Autodesk Inventor part; units mm, degrees
ref_plane "YZ Plane" through (0, 0, 0) normal (1, 0, 0) x (0, 1, 0)
ref_plane "XZ Plane" through (0, 0, 0) normal (0, 1, 0) x (-1, 0, 0)
ref_plane "XY Plane" through (0, 0, 0) normal (0, 0, 1) x (1, 0, 0)
sketch "Boceto1" plane through (0, 0, 0) normal (1, 0, 0) x (0, 1, 0)
  line L0 (0.5, 9) -> (-0.5, 9)
  line L1 (-0.5, 9) -> (-0.5, -9)
  line L2 (-0.5, -9) -> (0.5, -9)
  line L3 (0.5, -9) -> (0.5, 9)
  point P0 (0, 0)
  dimension "d0" = 1
  dimension "d1" = 18
  dimension "d2" = 9
  dimension "d3" = 0.5
extrude "Extrusión1" add sketch "Boceto1" along normal blind 50
sketch "Boceto2" plane through (0, 0.5, 9) normal (0, 1, 0) x (1, 0, 0)
  line L0 (0, 0) -> (50, 0)
  line L1 (0, 18) -> (50, 18)
  line L2 (0, 18) -> (0, 0)
  line L3 (25, 0) -> (25, 18)
  line L4 (0, 0) -> (50, 0)
  point P0 (0, 9)
  point P1 (2.54, 5.19)
  point P2 (2.54, 7.73)
  point P3 (2.54, 10.27)
  point P4 (2.54, 12.81)
  point P5 (47.46, 5.19)
  point P6 (47.46, 7.73)
  point P7 (47.46, 10.27)
  point P8 (47.46, 12.81)
  dimension "d6" = 5.19
  dimension "d8" = 2.54
  dimension "d9" = 2.54
  dimension "d10" = 2.54
  dimension "d11" = 2.54
hole "Agujero1" at (2.54, 0.5, 3.81) at (2.54, 0.5, 1.27) at (2.54, 0.5, -1.27) at (2.54, 0.5, -3.81) at (25, 0.5, 9) at (25, 0.5, -9) at (47.46, 0.5, -3.81) at (47.46, 0.5, -1.27) at (47.46, 0.5, 1.27) at (47.46, 0.5, 3.81) direction (0, -1, 0) diameter 0.9 end through all
sketch "Boceto3" plane through (0, 0.5, 9) normal (0, 1, 0) x (1, 0, 0)
  line L0 (37.0371, 5) -> (41.9064, 5)
  line L1 (41.9064, 5) -> (41.9064, 13)
  line L2 (41.9064, 13) -> (37.0371, 13)
  line L3 (37.0371, 13) -> (37.0371, 5)
  line L4 (25.45, 0) -> (50, 0)
  line L5 (25.45, 18) -> (50, 18)
  point P0 (0, 9)
  dimension "d19" = 5
  dimension "d20" = 5
extrude "Extrusión2" add sketch "Boceto3" along normal blind 5
properties part number "MAX485"
Build history of the part. All positions in model axes, mm. A direction names the side the tool comes from. Coordinates: 2 decimals unless noted, no trailing zeros. Order: outer loops, then holes, each group sorted by start corner. A loop starts at its lowest first (then second) coordinate and runs counter-clockwise, first axis right, second up. Notation, with made-up numbers: (-32.5, 50) - (17.5, 50) arc R11 ccw to (17.5, 62) - close; hole circle Ø8 at (19.5, 9.25). An arc over 180 degrees is marked (long way). Write each question's results on one line, items separated by ' | '. Start each with the question number.
Item 1: Band-saw the part on C-C on x = 37.5. Write the cut outline in (y, z).
Item 2: Band-saw the part on B-B on x = 47.46. Write the cut outline in (y, z), and give its area (3 significant figures).
Item 3: Mould opens along Z. For faces 1 (the face through (38, 0, 9)), 2 (the face through (12, 0, -9)), 3 (the face through (2.712, -0.007, -3.394)) say: released by +Z, released by -Z, zero draft, split by the parting line, or undercut.
Item 4: Band-saw the part on A-A on z = -1.27. Write the cut outline in (x, y).
Item 5: Tool access for faces 4 (the face through (41.906, 3, 0)), 5 (the face through (40, 3, -4)), 6 (the face through (39, 5.5, 0)), 7 (the face through (39, 3, 4)), 8 (the face through (2.712, -0.007, 4.226)): list every direction of +Z, -Z, +X, -X, +Y, -Y with a clear straight run to the whole face (end or side of a thin tool).
Item 6: Wall check: probe 1 along X at (y, z) = (0.1, 1.27); probe 2 along Z at (x, y) = (47.46, -0.1); probe 3 along X at (y, z) = (3.85, 2). Give the ranges that are in metal, low to high. Write a range as [from, to].
Item 7: Band-saw the part on D-D on z = 2.75. Write the cut outline in (x, y), and give its area (3 significant figures).
Item 8: Flat gauge pins, fed straight in: pin 1 (3 mm diameter, centred on y = 3.5, z = -2.5, fed in from +X); pin 2 (2.5 mm diameter, centred on y = 3, z = 0.5, fed in from -X); pin 3 (3 mm diameter, centred on x = 24.5, y = 1, fed in from +Z); pin 4 (2 mm diameter, centred on x = 12, z = -1.5, fed in from +Y). Where does each tip first touch, or does it go through?
Numbers:
1) outline: (-0.5, -9) - (0.5, -9) - (0.5, -4) - (5.5, -4) - (5.5, 4) - (0.5, 4) - (0.5, 9) - (-0.5, 9) - close
2) outline: (-0.5, -9) - (0.5, -9) - (0.5, -4.26) - (-0.5, -4.26) - close; (-0.5, -3.36) - (0.5, -3.36) - (0.5, -1.72) - (-0.5, -1.72) - close; (-0.5, -0.82) - (0.5, -0.82) - (0.5, 0.82) - (-0.5, 0.82) - close; (-0.5, 1.72) - (0.5, 1.72) - (0.5, 3.36) - (-0.5, 3.36) - close; (-0.5, 4.26) - (0.5, 4.26) - (0.5, 9) - (-0.5, 9) - close | area: 14.4 mm^2
3) face 1: released by +Z | face 2: released by -Z | face 3: undercut
4) outline: (0, -0.5) - (2.09, -0.5) - (2.09, 0.5) - (0, 0.5) - close; (2.99, -0.5) - (47.01, -0.5) - (47.01, 0.5) - (41.91, 0.5) - (41.91, 5.5) - (37.04, 5.5) - (37.04, 0.5) - (2.99, 0.5) - close; (47.91, -0.5) - (50, -0.5) - (50, 0.5) - (47.91, 0.5) - close
5) face 4: +Z, -Z, +X, +Y | face 5: -Z, +X, -X, +Y | face 6: +Z, -Z, +X, -X, +Y | face 7: +Z, +X, -X, +Y | face 8: +Y, -Y
6) probe 1: [0, 2.09], [2.99, 47.01], [47.91, 50] | probe 2: [-9, -4.26], [-3.36, -1.72], [-0.82, 0.82], [1.72, 3.36], [4.26, 9] | probe 3: [37.04, 41.91]
7) outline: (0, -0.5) - (50, -0.5) - (50, 0.5) - (41.91, 0.5) - (41.91, 5.5) - (37.04, 5.5) - (37.04, 0.5) - (0, 0.5) - close | area: 74.3 mm^2
8) pin 1: x = 41.91 | pin 2: x = 37.04 | pin 3: z = 9 | pin 4: y = 0.5
